Geometry: final body of the model. Coordinates: model frame, mm. A direction names the side the tool comes from. Coordinates: 2 decimals unless noted, no trailing zeros. Loops run counter-clockwise (first coordinate to the right, second up) from the corner with the lowest first, then second, coordinate; pieces in that order, holes last. Notation, with made-up numbers: (41, -22) - (99, -22) arc R10 ccw to (99, -13) - close; hole circle Ø6 at (77, 20). An arc over 180 degrees is marked (long way). Return JSON: item names as keys, results as strings.
from build123d import *

# Parameters (mm, degrees)
F1_DEPTH = 6.35


# Not quite as in the source:
# - ends of sketch curves that miss each other by under 0.0002 mm in the source are joined


with BuildPart() as f1:
    # F0 (on Front) → F1 (new body)
    with BuildSketch(Plane.XZ):
        with BuildLine():
            ThreePointArc((10.7423712, -19.0500001571), (13.9173712, -15.8750001571), (17.0923712, -19.0500001571))
            Line((17.0923712, -19.0500001571), (20.545679, -19.0500001571))
            Line((20.545679, -19.0500001571), (20.545679, -9.4996001571))
            Line((20.545679, -9.4996001571), (19.5523612, -9.4996001571))
            ThreePointArc((19.5523612, -9.4996001571), (17.3072971697, -8.5696641874), (16.3773612, -6.3246001571))
            Line((16.3773612, -6.3246001571), (16.3773612, 6.3245998429))
            ThreePointArc((16.3773612, 6.3245998429), (17.3072971697, 8.5696638731), (19.5523612, 9.4995998429))
            Line((19.5523612, 9.4995998429), (20.545679, 9.4995998429))
            Line((20.545679, 9.4995998429), (20.545679, 19.0499998429))
            Line((20.545679, 19.0499998429), (17.0923712, 19.0499998429))
            ThreePointArc((17.0923712, 19.0499998429), (13.9173712, 15.8749998429), (10.7423712, 19.0499998429))
            Line((10.7423712, 19.0499998429), (10.7423712, 25.3999998429))
            Line((10.7423712, 25.3999998429), (-10.7423712, 25.3999998429))
            Line((-10.7423712, 25.3999998429), (-10.7423712, 19.0499998429))
            ThreePointArc((-10.7423712, 19.0499998429), (-13.9173712, 15.8749998429), (-17.0923712, 19.0499998429))
            Line((-17.0923712, 19.0499998429), (-20.545679, 19.0499998429))
            Line((-20.545679, 19.0499998429), (-20.545679, 9.4995998429))
            Line((-20.545679, 9.4995998429), (-19.5523612, 9.4995998429))
            ThreePointArc((-19.5523612, 9.4995998429), (-17.3072971697, 8.5696638731), (-16.3773612, 6.3245998429))
            Line((-16.3773612, 6.3245998429), (-16.3773612, -6.3246001571))
            ThreePointArc((-16.3773612, -6.3246001571), (-17.3072971697, -8.5696641874), (-19.5523612, -9.4996001571))
            Line((-19.5523612, -9.4996001571), (-20.545679, -9.4996001571))
            Line((-20.545679, -9.4996001571), (-20.545679, -19.0500001571))
            Line((-20.545679, -19.0500001571), (-17.0923712, -19.0500001571))
            ThreePointArc((-17.0923712, -19.0500001571), (-13.9173712, -15.8750001571), (-10.7423712, -19.0500001571))
            Line((-10.7423712, -19.0500001571), (-10.7423712, -25.3999747571))
            Line((-10.7423712, -25.3999747571), (10.7423712, -25.3999747571))
            Line((10.7423712, -25.3999747571), (10.7423712, -19.0500001571))
        make_face()
        with BuildLine():
            Line((-7.5673712, 9.4996252429), (7.5673712, 9.4996252429))
            ThreePointArc((7.5673712, 9.4996252429), (9.8124352303, 8.5696638731), (10.7423712, 6.3245998429))
            Line((10.7423712, 6.3245998429), (10.7423712, -6.3246001571))
            ThreePointArc((10.7423712, -6.3246001571), (9.8124352303, -8.5696641874), (7.5673712, -9.4996001571))
            Line((7.5673712, -9.4996001571), (-7.5673712, -9.4996001571))
            ThreePointArc((-7.5673712, -9.4996001571), (-9.8124352303, -8.5696641874), (-10.7423712, -6.3246001571))
            Line((-10.7423712, -6.3246001571), (-10.7423712, 6.3245998429))
            ThreePointArc((-10.7423712, 6.3245998429), (-9.8124352303, 8.5696638731), (-7.5673712, 9.4996252429))
        make_face(mode=Mode.SUBTRACT)
    extrude(amount=F1_DEPTH)


solid = f1.part
Item 1: Ray query, probe 1 along Z at (x, y) = (-3, -2.75); probe 2 along X at (y, z) = (-3.25, -3); probe 3 along X at (y, z) = (-4, -18.5). Return the intervals inside material, ascending. Write a range as from..to.
Worked out:
{"probe 1": "-25.4..-9.5, 9.5..25.4", "probe 2": "-16.38..-10.74, 10.74..16.38", "probe 3": "-20.55..-17.04, -10.79..10.79, 17.04..20.55"}
Item 2: Mould query, pull axis X, two halves, no side actions, for faces 1 (the face through (13.848, -3.131, -15.876)), 2 (the face through (10.742, -3, 22)), 3 (the face through (0, -3, -25.4)). Classes: +X half, -X half, draft (parallel to the pull), parting line (faces both ways), or undercut.
Worked out:
{"face 1": "undercut", "face 2": "+X half", "face 3": "draft"}
Item 3: Reachability of faces 4 (the face through (-17.33, -3.13, 8.59)), 5 (the face through (-10.742, -3, -22)), 6 (the face through (-9.79, -3.13, -8.59)) from +Z, -Z, +X, -X, +Y, -Y: full face, straight path, thin tool, end or side. Return the list, or none.
Worked out:
{"face 4": "-X, +Y, -Y", "face 5": "-Z, -X, +Y, -Y", "face 6": "+Y, -Y"}
Item 4: Section query D-D, the plane x = 14.5. Return loops of the section in (y, z), and give its area (3 significant figures).
Worked out:
{"outline": "(-6.35, -15.93) - (0, -15.93) - (0, 15.93) - (-6.35, 15.93) - close", "area": "202 mm^2"}
Item 5: First-contact query: pin 1 Ø1 at (x, y) = (13, -3) entering from +Z; pin 2 Ø1.9 at (y, z) = (-2.5, 0) entering from -X; pin 3 Ø0.5 at (x, y) = (20, -3) entering from +Z. Flat tips, straight axial feed; report the tip coordinate or a pass-through.
Worked out:
{"pin 1": "z = 16.21", "pin 2": "x = -16.38", "pin 3": "z = 19.05"}
Item 6: Section query B-B, the plane z = -3. Return loops of the section in (x, y), and give its area (3 significant figures).
Worked out:
{"outline": "(-16.38, -6.35) - (-10.74, -6.35) - (-10.74, 0) - (-16.38, 0) - close; (10.74, -6.35) - (16.38, -6.35) - (16.38, 0) - (10.74, 0) - close", "area": "71.6 mm^2"}
Item 7: Section query C-C, the plane z = -17. Return loops of the section in (x, y), and give its area (3 significant figures).
Worked out:
{"outline": "(-20.55, -6.35) - (-16.34, -6.35) - (-16.34, 0) - (-20.55, 0) - close; (-11.49, -6.35) - (11.49, -6.35) - (11.49, 0) - (-11.49, 0) - close; (16.34, -6.35) - (20.55, -6.35) - (20.55, 0) - (16.34, 0) - close", "area": "199 mm^2"}
Item 8: Section query A-A, the plane x = 6. Return loops of the section in (y, z), and give its area (3 significant figures).
Worked out:
{"outline": "(-6.35, -25.4) - (0, -25.4) - (0, -9.5) - (-6.35, -9.5) - close; (-6.35, 9.5) - (0, 9.5) - (0, 25.4) - (-6.35, 25.4) - close", "area": "202 mm^2"}
